from build123d import *

# Parameters (mm, degrees)
SKETCH1_R               = 1.35
BOSS_EXTRUDE1_DEPTH     = 9
SKETCH2_R               = 2.5
SKETCH2_R_2             = 1.9
BOSS_EXTRUDE2_DEPTH     = 6.5
CRVPATTERN1_START       = 9
CRVPATTERN1_OUTLINE_R   = 2.5
CRVPATTERN1_OUTLINE_R_2 = 1.9
CRVPATTERN1_DEPTH       = 6.5


# Read off the part's stored shape, not the designer's step: CrvPattern1
with BuildPart() as part:
    # Sketch1 → Boss-Extrude1 (new body)
    with BuildSketch(Plane.XY):
        with BuildLine():
            Line((11.25, 8.1), (11.25, -8.1))
            Line((11.25, -8.1), (5.25, -8.1))
            Line((5.25, -8.1), (5.25, -2.618563538))
            ThreePointArc((5.25, -2.618563538), (4.125, -2.85), (3, -2.618563538))
            Line((3, -2.618563538), (3, -8.1))
            Line((3, -8.1), (-3, -8.1))
            Line((-3, -8.1), (-3, -2.618563538))
            ThreePointArc((-3, -2.618563538), (-4.125, -2.85), (-5.25, -2.618563538))
            Line((-5.25, -2.618563538), (-5.25, -8.1))
            Line((-5.25, -8.1), (-11.25, -8.1))
            Line((-11.25, -8.1), (-11.25, 8.1))
            Line((-11.25, 8.1), (-5.25, 8.1))
            Line((-5.25, 8.1), (-5.25, 2.618563538))
            ThreePointArc((-5.25, 2.618563538), (-4.125, 2.85), (-3, 2.618563538))
            Line((-3, 2.618563538), (-3, 8.1))
            Line((-3, 8.1), (3, 8.1))
            Line((3, 8.1), (3, 2.618563538))
            ThreePointArc((3, 2.618563538), (4.125, 2.85), (5.25, 2.618563538))
            Line((5.25, 2.618563538), (5.25, 8.1))
            Line((5.25, 8.1), (11.25, 8.1))
        make_face()
        with Locations((-4.125, 0)):
            Circle(SKETCH1_R, mode=Mode.SUBTRACT)
        with Locations((4.125, 0)):
            Circle(SKETCH1_R, mode=Mode.SUBTRACT)
    extrude(amount=BOSS_EXTRUDE1_DEPTH)

    # Sketch2 → Boss-Extrude2 (add)
    with BuildSketch(Plane.XY.offset(9)):
        with Locations(Location((0, 4.25, 0), (0, 0, 180))):
            Circle(SKETCH2_R)
        with Locations(Location((0, 4.25, 0), (0, 0, 180))):
            Circle(SKETCH2_R_2, mode=Mode.SUBTRACT)
    boss_extrude2 = extrude(amount=BOSS_EXTRUDE2_DEPTH)

    # CrvPattern1 outline → CrvPattern1 (add)
    # profile 1 of 2: a face of its own
    with BuildSketch(Plane.XY.offset(CRVPATTERN1_START)):
        with Locations((8.25, 4.25)):
            Circle(CRVPATTERN1_OUTLINE_R)
        with Locations((8.25, 4.25)):
            Circle(CRVPATTERN1_OUTLINE_R_2, mode=Mode.SUBTRACT)
    # profile 2 of 2: a face of its own
    with BuildSketch(Plane.XY.offset(CRVPATTERN1_START)):
        with Locations((-8.25, 4.25)):
            Circle(CRVPATTERN1_OUTLINE_R)
        with Locations((-8.25, 4.25)):
            Circle(CRVPATTERN1_OUTLINE_R_2, mode=Mode.SUBTRACT)
    crvpattern1 = extrude(amount=CRVPATTERN1_DEPTH)

    # Mirror1: Boss-Extrude2, CrvPattern1 across plane
    add(boss_extrude2.mirror(Plane.ZX))
    add(crvpattern1.mirror(Plane.ZX))


solid = part.part
Can you work these out from the model? Positions are in its coordinate system, mm. A direction names the side the tool comes from. Give positions to 0.01 mm unless a question says otherwise; leave off trailing zeros. Write each loop counter-clockwise with the first axis right and the second up, starting at its lowest first coordinate (ties: lowest second). Pieces come first, ordered by that corner, then holes. Notation, with made-up numbers: M 81.25,8.25 L 90.25,8.25 A21 cw 90.25,43.25 Z; hole C -26,81.25 d4. An arc over 180 degrees is marked long. Answer in a Markdown table with one row per item. Add a question column.
Item 1: Imagine slicing it at D-D, the plane x = -4.25. Write out the boundary of the cut face in (y, z), plus the area to 3 significant figures.
Item 2: Imagine slicing it at B-B, the plane y = 0. Write out the boundary of the cut face in (x, z) (3 decimals).
Item 3: On a 3-axis mill with a long thin cutter (end or side, diameter ignored), from which of +Z, -Z, +X, -X, +Y, -Y can I reach the whole of each face in a straight line? I mean faces 5 (the cylindrical face through (0.33, 1.77, 12.2)), 6 (the flat face through (-5.25, -5, 4)), 7 (the flat face through (-8, -8.1, 4)). Say none if no direction works.
Item 4: Please list where these lines run through material, in increasing order: L1, parallel to Y at x = -8.25, z = 13.25; L2, parallel to X at y = -4, z = 4; L3, parallel to Y at x = -4.25, z = 5.
Item 5: We'd pull the mould along X, two halves only. Please class faces 1 (the flat face through (-10, 3, 15.5)), 2 (the cylindrical face through (10.635, 5.001, 12.204)), 3 (the cylindrical face through (4.14, -2.85, 4.44)), 4 (the flat face through (11.25, 0, 4)): released by +X, released by -X, zero draft, split by the parting line, or undercut.
Item 6: Imagine slicing it at C-C, the plane z = 8. Write out the boundary of the cut face in (x, y) (3 decimals), plus the area to 3 significant figures.
Item 7: Imagine slicing it at A-A, the plane z = 13.75. State how many separate pieces and enclosed holes the cut face has, plus the area to 3 significant figures.
Item 8: For pin 1 Ø3.5 at (x, y) = (-8.25, 4.25) entering from +Z; pin 2 Ø5 at (x, z) = (7, 13.5) entering from -Y, each with a flat end and sliding along its axis, tell me the tip position at first contact or that it passes through.
Evaluation:
| question | item | result |
|---|---|---|
| 1 | outline | M -2.85,0 L -1.34,0 L -1.34,9 L -2.85,9 Z; M 1.34,0 L 2.85,0 L 2.85,9 L 1.34,9 Z |
| 1 | area | 27.1 mm² |
| 2 | outline | M -11.25,0 L -5.475,0 L -5.475,9 L -11.25,9 Z; M -2.775,0 L 2.775,0 L 2.775,9 L -2.775,9 Z; M 5.475,0 L 11.25,0 L 11.25,9 L 5.475,9 Z |
| 3 | face 5 | +Z |
| 3 | face 6 | +Z, -Z, -Y |
| 3 | face 7 | +Z, -Z, +X, -X, -Y |
| 4 | L1 | y = -6.75 to -6.15, -2.35 to -1.75, 1.75 to 2.35, 6.15 to 6.75 |
| 4 | L2 | x = -11.25 to -5.25, -3 to 3, 5.25 to 11.25 |
| 4 | L3 | y = -2.85 to -1.34, 1.34 to 2.85 |
| 5 | face 1 | zero draft |
| 5 | face 2 | undercut |
| 5 | face 3 | undercut |
| 5 | face 4 | released by +X |
| 6 | outline | M -11.25,-8.1 L -5.25,-8.1 L -5.25,-2.619 A2.85 ccw -3,-2.619 L -3,-8.1 L 3,-8.1 L 3,-2.619 A2.85 ccw 5.25,-2.619 L 5.25,-8.1 L 11.25,-8.1 L 11.25,8.1 L 5.25,8.1 L 5.25,2.619 A2.85 ccw 3,2.619 L 3,8.1 L -3,8.1 L -3,2.619 A2.85 ccw -5.25,2.619 L -5.25,8.1 L -11.25,8.1 Z; hole C -4.125,0 d2.7; hole C 4.125,0 d2.7 |
| 6 | area | 305 mm² |
| 7 | separate pieces | 6 |
| 7 | enclosed holes | 6 |
| 7 | area | 49.8 mm² |
| 8 | pin 1 | stops at z = 9 |
| 8 | pin 2 | stops at y = -6.75 |
